from build123d import *

# Parameters (mm, degrees)
ESQUISSE1_R                  = 19.24
BOSS_EXTRU_1_DEPTH           = 5
ESQUISSE2_R                  = 0.53
ENL_V_MAT_EXTRU_1_DEPTH      = 5
R_P_TITION_CIRCULAIRE1_COUNT = 4


with BuildPart() as part:
    # Esquisse1 → Boss.-Extru.1 (new body)
    with BuildSketch(Plane.XY):
        Circle(ESQUISSE1_R)
    extrude(amount=BOSS_EXTRU_1_DEPTH)

    # Esquisse2 → Enlèv. mat.-Extru.1 (cut)
    with BuildSketch(Plane.XY.offset(5)):
        with Locations((0, 8.06)):
            Circle(ESQUISSE2_R)
    enl_v_mat_extru_1 = extrude(amount=-ENL_V_MAT_EXTRU_1_DEPTH, mode=Mode.SUBTRACT)

    # Répétition circulaire1: Enlèv. mat.-Extru.1 ×4 about axis
    r_p_tition_circulaire1_axis = Axis((0, 0, 0), (0, 0, 1))
    for i in range(1, R_P_TITION_CIRCULAIRE1_COUNT):
        add(enl_v_mat_extru_1.rotate(r_p_tition_circulaire1_axis, i * 360 / R_P_TITION_CIRCULAIRE1_COUNT), mode=Mode.SUBTRACT)


solid = part.part
Can you work these out from the model? Positions are in its coordinate system, mm. Round coordinates to 2 decimals unless told otherwise and drop trailing zeros. Loops run counter-clockwise (first coordinate to the right, second up) from the corner with the lowest first, then second, coordinate; pieces in that order, holes last. Notation, with made-up numbers: (-32, 11) - (24, 11) arc R28 ccw to (24, 49) - close; hole circle Ø1 at (39, -16.75). An arc over 180 degrees is marked (long way). Answer in a Markdown table with one row per item. Add a question column.
Q1. I want a section at D-D on y = -8.06. List the corners of the cut face in (x, z) for me, and give its area (3 significant figures).
Q2. I want a section at C-C on z = 3.6. List the corners of the cut face in (x, y) for me.
Q3. For pin 1 Ø1 at (x, y) = (8.06, 0) entering from +Z; pin 2 Ø1 at (y, z) = (2.5, 3.5) entering from -X; pin 3 Ø2 at (x, z) = (-14, 4) entering from -Y, each with a flat end and sliding along its axis, tell me the tip position at first contact or that it passes through.
Q4. I need wall thicknesses on L1, parallel to Y at x = 0, z = 3; L2, parallel to X at y = -8.06, z = 2.65; L3, parallel to X at y = -8.5, z = 2.35. Which ranges of each line are inside material? Lowest first, please.
Q5. I want a section at A-A on y = 0. List the corners of the cut face in (x, z) for me, and give its area (3 significant figures).
Q6. We'd pull the mould along Y, two halves only. Please class faces 1 (the cylindrical face through (0.11, -7.54, 2.54)), 2 (the cylindrical face through (-19.22, 0.85, 2.46)), 3 (the flat face through (0, 0, 0)): pulls with the +Y half, pulls with the -Y half, needs draft (parallel to the pull), parting line crosses it, or undercut.
A:
| question | item | result |
|---|---|---|
| 1 | outline | (-17.47, 0) - (-0.53, 0) - (-0.53, 5) - (-17.47, 5) - close; (0.53, 0) - (17.47, 0) - (17.47, 5) - (0.53, 5) - close |
| 1 | area | 169 mm^2 |
| 2 | outline | circle Ø38.48 at (0, 0); hole circle Ø1.06 at (-8.06, 0); hole circle Ø1.06 at (0, -8.06); hole circle Ø1.06 at (0, 8.06); hole circle Ø1.06 at (8.06, 0) |
| 3 | pin 1 | through |
| 3 | pin 2 | x = -19.14 |
| 3 | pin 3 | y = -14.18 |
| 4 | L1 | -19.24 to -8.59, -7.53 to 7.53, 8.59 to 19.24 |
| 4 | L2 | -17.47 to -0.53, 0.53 to 17.47 |
| 4 | L3 | -17.26 to -0.3, 0.3 to 17.26 |
| 5 | outline | (-19.24, 0) - (-8.59, 0) - (-8.59, 5) - (-19.24, 5) - close; (-7.53, 0) - (7.53, 0) - (7.53, 5) - (-7.53, 5) - close; (8.59, 0) - (19.24, 0) - (19.24, 5) - (8.59, 5) - close |
| 5 | area | 182 mm^2 |
| 6 | face 1 | undercut |
| 6 | face 2 | parting line crosses it |
| 6 | face 3 | needs draft |
